Verification items for the finished model (mm, model axes). A direction names the side the tool comes from. Coordinates: 2 decimals unless noted, no trailing zeros. Loops run counter-clockwise (first coordinate to the right, second up) from the corner with the lowest first, then second, coordinate; pieces in that order, holes last. Notation, with made-up numbers: (53, 47.5) - (69, 47.5) arc R11 ccw to (69, 63.5) - close; hole circle Ø10 at (-5, 4.5). An arc over 180 degrees is marked (long way). One line per item, written item: value. Start each with the question number.
(1) Draft check along Y on faces 1 (the face through (-29, -11.347, 10)), 2 (the face through (-33.773, 11.343, 9.087)), 3 (the face through (-29.083, 12, 10)). Enter one of: +Y half, -Y half, draft (parallel to the pull), parting line (faces both ways), or undercut.
(2) Section check B-B (z = 2.5). Record the boundary of the cut face in (x, y) (1 decimal).
(3) Thickness scan on probe 1 along Y at (x, z) = (-35.5, 8.75); probe 2 along Y at (x, z) = (-39.5, 7.5); probe 3 along X at (y, z) = (10.25, 1.5). Record the ranges inside material, lowest first. Write a range as [from, to].
(4) Section check A-A (y = 10). Record the boundary of the cut face in (x, z).
(5) Set-up check for faces 4 (the face through (-38.333, 4, 10)), 5 (the face through (-13.3, -5.347, 7.6)), 6 (the face through (-22.133, 9.1, 8.6)), 7 (the face through (-44.54, -8.31, 11.9)), 8 (the face through (-33, -7, 20)): record each of +Z, -Z, +X, -X, +Y, -Y from which the full face is reachable in a straight line by a thin tool's end or side.
(6) Section check C-C (z = 10). Count the separate pieces of the cut face and the enclosed holes in it, plus the area to 3 significant figures.
(7) Gauge pin test, flat ends, axial feed: P1, Ø8, axis at y = 4, z = 3.5, coming from the +X side; P2, Ø0.8, axis at x = -20.5, z = 11.5, coming from the +Y side; P3, Ø3, axis at x = -41.5, z = 11, coming from the +Y side. Record the tip position at first contact, or that the pin passes through.
```python
from build123d import *

# Parameters (mm, degrees)
F1_DEPTH = 20
F2_R     = 1.5
F3_DEPTH = 20
F4_W     = 2.8
F4_H     = 6
F5_DEPTH = 7.5
F6_R     = 2.25
F7_DEPTH = 6


with BuildPart() as f1:
    # F0 (on Top) → F1 (new body)
    with BuildSketch(Plane.XY):
        with BuildLine():
            Line((-38.333333, 13.652778), (-38.333333, -5.347222))
            Line((-38.333333, -5.347222), (-34.498064, -5.347222))
            ThreePointArc((-34.498064, -5.347222), (-35.652397, 2.724457), (-29.083333, 7.554765))
            Line((-29.083333, 7.554765), (-29.083333, 13.652778))
            Line((-29.083333, 13.652778), (-38.333333, 13.652778))
        make_face()
        with BuildLine():
            Line((-48.333333, -5.347222), (-48.333333, -11.347222))
            Line((-48.333333, -11.347222), (-8.333333, -11.347222))
            Line((-8.333333, -11.347222), (-8.333333, -5.347222))
            Line((-8.333333, -5.347222), (-18.333333, -5.347222))
            Line((-18.333333, -5.347222), (-22.168602, -5.347222))
            ThreePointArc((-22.168602, -5.347222), (-28.333333, -8.284722), (-34.498064, -5.347222))
            Line((-34.498064, -5.347222), (-38.333333, -5.347222))
            Line((-38.333333, -5.347222), (-48.333333, -5.347222))
        make_face()
        with BuildLine():
            Line((-22.168602, -5.347222), (-18.333333, -5.347222))
            Line((-18.333333, -5.347222), (-18.333333, 13.652778))
            Line((-18.333333, 13.652778), (-27.583333, 13.652778))
            Line((-27.583333, 13.652778), (-27.583333, 7.554765))
            ThreePointArc((-27.583333, 7.554765), (-22.461492, 4.993694), (-20.395833, -0.347222))
            ThreePointArc((-20.395833, -0.347222), (-20.852142, -2.999707), (-22.168602, -5.347222))
        make_face()
    extrude(amount=F1_DEPTH)

    # F2 (on face) → F3 (cut)
    with BuildSketch(Plane(origin=(-38.333333, 0, 0), x_dir=(0, -1, 0), z_dir=(-1, 0, 0))):
        with Locations((-10.152778, 10)):
            Circle(F2_R)
    extrude(amount=-F3_DEPTH, mode=Mode.SUBTRACT)

    # F4 (on face) → F5 (cut)
    with BuildSketch(Plane(origin=(0, 13.652778, 0), x_dir=(-1, 0, 0), z_dir=(0, 1, 0))):
        with Locations((20.733333, 10)):
            Rectangle(F4_W, F4_H)
    extrude(amount=-F5_DEPTH, mode=Mode.SUBTRACT)

    # F6 (on face) → F7 (cut)
    with BuildSketch(Plane(origin=(0, -5.347222, 0), x_dir=(-1, 0, 0), z_dir=(0, 1, 0))):
        with Locations((43.333333, 10)):
            Circle(F6_R)
        with Locations((13.333333, 10)):
            Circle(F6_R)
    extrude(amount=-F7_DEPTH, mode=Mode.SUBTRACT)


solid = f1.part
```
Responses:
1. face 1: -Y half
1. face 2: undercut
1. face 3: draft
2. outline: (-48.3, -11.3) - (-8.3, -11.3) - (-8.3, -5.3) - (-18.3, -5.3) - (-18.3, 13.7) - (-27.6, 13.7) - (-27.6, 7.6) arc R7.9 cw to (-20.4, -0.3) arc R7.9 cw to (-22.2, -5.3) arc R7.9 cw (long way) to (-29.1, 7.6) - (-29.1, 13.7) - (-38.3, 13.7) - (-38.3, -5.3) - (-48.3, -5.3) - close
3. probe 1: y = [-11.35, -3.76], [3.06, 9.32], [10.98, 13.65]
3. probe 2: y = [-11.35, -5.35]
3. probe 3: x = [-38.33, -29.08], [-27.58, -18.33]
4. outline: (-38.33, 0) - (-29.08, 0) - (-29.08, 8.51) - (-38.33, 8.51) - close; (-38.33, 11.49) - (-29.08, 11.49) - (-29.08, 20) - (-38.33, 20) - close; (-27.58, 0) - (-18.33, 0) - (-18.33, 8.51) - (-19.33, 8.51) - (-19.33, 7) - (-22.13, 7) - (-22.13, 8.51) - (-27.58, 8.51) - close; (-27.58, 11.49) - (-22.13, 11.49) - (-22.13, 13) - (-19.33, 13) - (-19.33, 11.49) - (-18.33, 11.49) - (-18.33, 20) - (-27.58, 20) - close
5. face 4: +Z, -Z, -X, +Y
5. face 5: +Z, -Z, +X, +Y
5. face 6: +Y
5. face 7: +Y, -Y
5. face 8: +Z, +X, -X, +Y, -Y
6. separate pieces: 6
6. enclosed holes: 0
6. area: 291 mm²
7. P1: stops at x = -18.33
7. P2: stops at y = 6.15
7. P3: stops at y = -5.35
